from build123d import *

# Parameters (mm, degrees)
SKETCH1_R           = 2.5
SKETCH1_W           = 40
SKETCH1_H           = 20
BOSS_EXTRUDE1_DEPTH = 3.175


with BuildPart() as part:
    # Sketch1 → Boss-Extrude1 (new body)
    with BuildSketch(Plane.XY):
        Polygon((-101.6, 0), (-83.3, 0), (-83.3, 3.175), (-78.3, 3.175), (-78.3, 0), (-73.3, 0), (-73.3, 3.175), (-68.3, 3.175), (-68.3, 0), (-63.3, 0), (-63.3, 3.175), (-58.3, 3.175), (-58.3, 0), (-53.3, 0), (-53.3, 3.175), (-48.3, 3.175), (-48.3, 0), (-43.3, 0), (-43.3, 3.175), (-38.3, 3.175), (-38.3, 0), (-33.3, 0), (-33.3, 3.175), (-28.3, 3.175), (-28.3, 0), (-23.3, 0), (-23.3, 3.175), (-18.3, 3.175), (-18.3, 0), (0, 0), (0, -5), (3.175, -5), (3.175, -10), (0, -10), (0, -15), (3.175, -15), (3.175, -20), (0, -20), (0, -25), (3.175, -25), (3.175, -30), (0, -30), (0, -38.1), (-101.6, -38.1), (-101.6, -30), (-104.775, -30), (-104.775, -25), (-101.6, -25), (-101.6, -20), (-104.775, -20), (-104.775, -15), (-101.6, -15), (-101.6, -10), (-104.775, -10), (-104.775, -5), (-101.6, -5), align=None)
        with Locations((-25.4, -25.4)):
            Circle(SKETCH1_R, mode=Mode.SUBTRACT)
        with Locations((-66.2, -25.4)):
            Rectangle(SKETCH1_W, SKETCH1_H, mode=Mode.SUBTRACT)
    extrude(amount=BOSS_EXTRUDE1_DEPTH)


solid = part.part
For this review, take the finished solid that the model builds, in its own axes (mm). A direction names the side the tool comes from. Round coordinates to 2 decimals unless told otherwise and drop trailing zeros. Write each loop counter-clockwise with the first axis right and the second up, starting at its lowest first coordinate (ties: lowest second). Pieces come first, ordered by that corner, then holes. Notation, with made-up numbers: (36.25, 2.5) -> (90.25, 2.5) arc R19 ccw to (90.25, 24.5) -> close; hole circle Ø9 at (85.5, 27.25). An arc over 180 degrees is marked (long way). Put each result on its own line as item: value.
Q1. Clearance check with flat-ended pins moving along their axes: pin 1 Ø1.6 at (x, z) = (1.5, 2) entering from -Y; pin 2 Ø1.5 at (y, z) = (-12.5, 1.5) entering from +X; pin 3 Ø1 at (x, z) = (-103.5, 1) entering from +Y; pin 4 Ø8 at (x, y) = (-72.5, -30) entering from +Z. State where each tip first meets the part, or that it passes through.
Determined:
pin 1: stops at y = -30
pin 2: stops at x = 0
pin 3: stops at y = -5
pin 4: passes through
Q2. Consider section B-B on x = -50.5. State the section outline as (y, z) points (3 decimals), and give its area (3 significant figures).
Determined:
outline: (-38.1, 0) -> (-35.4, 0) -> (-35.4, 3.175) -> (-38.1, 3.175) -> close; (-15.4, 0) -> (3.175, 0) -> (3.175, 3.175) -> (-15.4, 3.175) -> close
area: 67.5 mm^2
Q3. Consider section D-D on x = -95.5. State the section outline as (y, z) points (3 decimals), and give its area (3 significant figures).
Determined:
outline: (-38.1, 0) -> (0, 0) -> (0, 3.175) -> (-38.1, 3.175) -> close
area: 121 mm^2
Q4. To check wall thickness, follow L1, parallel to X at y = -17, z = 0.7 (3 decimals); L2, parallel to Y at x = -25.4, z = 1.75; L3, parallel to Y at x = -69.5, z = 1.4 (3 decimals). State the ranges of each line that lie inside material, in increasing order. Write a range as [from, to].
Determined:
L1: x = [-104.775, -86.2], [-46.2, 3.175]
L2: y = [-38.1, -27.9], [-22.9, 0]
L3: y = [-38.1, -35.4], [-15.4, 3.175]
Q5. The part is to be moulded in two halves that separate along Y. For faces 6 (the flat face through (-46, 0, 2)), 7 (the flat face through (-50, -13, 3.175)), 8 (the flat face through (-101.6, -23, 2)), say which applies: released by +Y, released by -Y, zero draft, split by the parting line, or undercut.
Determined:
face 6: released by +Y
face 7: zero draft
face 8: undercut
Q6. Consider section A-A on x = -25.4. State the section outline as (y, z) points (3 decimals), and give its area (3 significant figures).
Determined:
outline: (-38.1, 0) -> (-27.9, 0) -> (-27.9, 3.175) -> (-38.1, 3.175) -> close; (-22.9, 0) -> (0, 0) -> (0, 3.175) -> (-22.9, 3.175) -> close
area: 105 mm^2
Q7. Consider section C-C on z = 1.75. Give the number of separate pieces and of enclosed holes in the cut face, and give its area (3 significant figures).
Determined:
separate pieces: 1
enclosed holes: 2
area: 3,260 mm^2
Q8. Machinability: for faces 1 (the flat face through (-103, -15, 2)), 2 (the flat face through (0, -12, 2)), 3 (the flat face through (-103, -5, 2)), 4 (the flat face through (-104.775, -8, 2)), 5 (the flat face through (-38.3, 2, 2)), which of the approach directions +Z, -Z, +X, -X, +Y, -Y give a long, thin tool a straight path to every point of the face, cutting with its end or side? Answer none if there is none.
Determined:
face 1: +Z, -Z, -X
face 2: +Z, -Z, +X
face 3: +Z, -Z, -X, +Y
face 4: +Z, -Z, -X, +Y, -Y
face 5: +Z, -Z, +Y
